```python
from build123d import *

# Parameters (mm, degrees)
F0_R     = 25.4
F1_DEPTH = 31.75
F2_R     = 15.875
F3_DEPTH = 28.575
F4_R     = 12.7
F5_DEPTH = 60.325


with BuildPart() as f1:
    # F0 (on Front) → F1 (new body)
    with BuildSketch(Plane.XZ):
        Circle(F0_R)
    extrude(amount=-F1_DEPTH)

    # F2 (on face) → F3 (join)
    with BuildSketch(Plane.XZ):
        Circle(F2_R)
    extrude(amount=F3_DEPTH)

    # F4 (on face) → F5 (cut)
    with BuildSketch(Plane.XZ.offset(28.575)):
        Circle(F4_R)
    extrude(amount=-F5_DEPTH, mode=Mode.SUBTRACT)


solid = f1.part
```
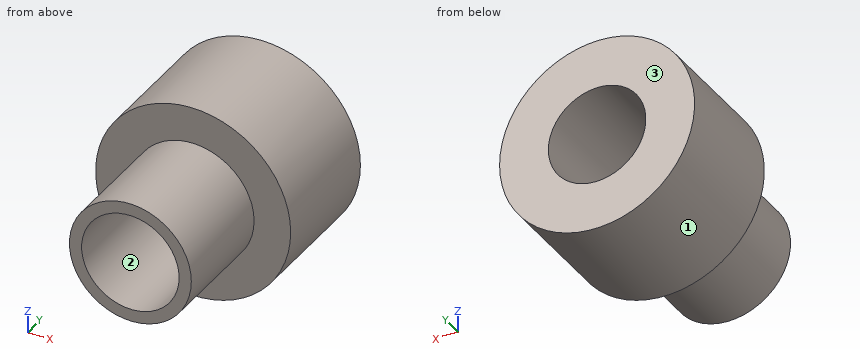
Design review of the part built by this model. Coordinates are the model's own, in mm. Face numbers are marked on the shaded views. Coordinates: 2 decimals unless noted, no trailing zeros. Write each loop counter-clockwise with the first axis right and the second up, starting at its lowest first coordinate (ties: lowest second). Pieces come first, ordered by that corner, then holes.
1) Insertion check: pin 1 (10 mm diameter, centred on x = -15.5, y = -20, fed in from +Z); pin 2 (12 mm diameter, centred on y = 21.5, z = -6.5, fed in from -X); pin 3 (2 mm diameter, centred on y = 7.5, z = -5.5, fed in from +X). Each pin has a flat end and moves straight along its axis. Give the tip position at first contact, or say it passes through.
2) Add section D-D (x = -20). Write out the cut boundary in (y, z), plus the area to 3 significant figures.
3) Mouldability with a two-part tool opening along Z and no side actions: class the marked faces 1, 2 and 3 as +Z half, -Z half, draft (parallel to the pull), parting line (faces both ways), or undercut.
4) Add section B-B (x = 0). Write out the cut boundary in (y, z) (3 decimals).
5) Add section C-C (y = 20). Write out the cut boundary in (x, z), plus the area to 3 significant figures.
6) Add section A-A (z = 0). Write out the cut boundary in (x, y) (3 decimals).
7) To check wall thickness, follow L1, parallel to Z at x = 0, y = 27; L2, parallel to Z at x = 0, y = -11 (3 decimals); L3, parallel to Y at x = 8.5, z = -18. State the ranges of each line that lie inside material, in increasing order.
Check result:
1. pin 1: stops at z = 11.91
1. pin 2: stops at x = -25.4
1. pin 3: stops at x = 25
2. outline: (0, -15.66) - (31.75, -15.66) - (31.75, 15.66) - (0, 15.66) - close
2. area: 994 mm2
3. face 1: parting line
3. face 2: undercut
3. face 3: draft
4. outline: (-28.575, -15.875) - (0, -15.875) - (0, -25.4) - (31.75, -25.4) - (31.75, -12.7) - (-28.575, -12.7) - close; (-28.575, 12.7) - (31.75, 12.7) - (31.75, 25.4) - (0, 25.4) - (0, 15.875) - (-28.575, 15.875) - close
5. outline: circle Ø50.8 at (0, 0); hole circle Ø25.4 at (0, 0)
5. area: 1,520 mm2
6. outline: (-25.4, 0) - (-15.875, 0) - (-15.875, -28.575) - (-12.7, -28.575) - (-12.7, 31.75) - (-25.4, 31.75) - close; (12.7, -28.575) - (15.875, -28.575) - (15.875, 0) - (25.4, 0) - (25.4, 31.75) - (12.7, 31.75) - close
7. L1: z = -25.4 to -12.7, 12.7 to 25.4
7. L2: z = -15.875 to -12.7, 12.7 to 15.875
7. L3: y = 0 to 31.75
